```python
from build123d import *

# Parameters (mm, degrees)
F2_R           = 12.6873
F3_DEPTH       = 1.524
F4_R           = 10.16
F5_DEPTH       = 25.4
F7_ANGLE       = 10
F8_W           = 12.7
F8_H           = 2.5441443902
F9_ANGLE_BACK  = 5
F9_ANGLE       = 20
F10_W          = 12.7
F10_H          = 2.5441443902
F11_ANGLE_BACK = 5
F11_ANGLE      = 20


with BuildPart() as f1:
    # F0 (on Front) → F1 (revolve)
    with BuildSketch(Plane.XZ):
        with BuildLine():
            Line((-13.97, 0), (-12.7, 0))
            Line((-12.7, 0), (-12.7, 5.76834))
            ThreePointArc((-12.7, 5.76834), (-12.5140128061, 6.2173528061), (-12.065, 6.40334))
            Line((-12.065, 6.40334), (0, 6.40334))
            Line((0, 6.40334), (0, 8.43534))
            Line((0, 8.43534), (-12.0142573769, 8.43534))
            ThreePointArc((-12.0142573769, 8.43534), (-13.3560582498, 7.8825956776), (-13.9192, 6.5451252153))
            Line((-13.9192, 6.5451252153), (-13.97, 0))
        make_face()
    revolve(axis=Axis((0, 0, 7.41934), (0, 0, 1)))

    # F2 (on face) → F3 (cut)
    with BuildSketch(Plane.XY.offset(8.43534)):
        Circle(F2_R)
    extrude(amount=-F3_DEPTH, mode=Mode.SUBTRACT)

    # F4 (on face) → F5 (cut)
    with BuildSketch(Plane.XY.offset(6.91134)):
        Circle(F4_R)
    extrude(amount=-F5_DEPTH, mode=Mode.SUBTRACT)

    # F6 (on Right) → F7 (revolve)
    with BuildSketch(Plane.YZ):
        with BuildLine():
            add(Edge.make_bspline(
                [(-12.7, 2.54), (-12.3650313684, 2.0936619038), (-12.0236620945, 1.3279431517), (-12.3556444426, 0.3304517928), (-12.7, 0)],
                knots=[0, 0, 0, 0, 0.5, 1, 1, 1, 1], degree=3))
            Line((-12.7, 2.54), (-12.7, 0))
        make_face()
        with BuildLine():
            Line((12.7, 0), (12.7, 2.54))
            add(Edge.make_bspline(
                [(12.7, 2.54), (12.4156702788, 2.2468428115), (11.9749216364, 1.2698282605), (12.4024864485, 0.2935006674), (12.7, 0)],
                knots=[0, 0, 0, 0, 0.5, 1, 1, 1, 1], degree=3))
        make_face()
    revolve(axis=Axis((0, 0, 2.8421400978), (0, 0, 1)), revolution_arc=F7_ANGLE)

    # F8 (on Right) → F9 (revolve, cut)
    with BuildSketch(Plane.YZ, mode=Mode.PRIVATE) as f9_sk:
        with Locations((6.35, 7.0404121951)):
            Rectangle(F8_W, F8_H)
    revolve(f9_sk.sketch.rotate(Axis((0, 0, 7.0404121951), (0, 0, 1)), -F9_ANGLE_BACK), axis=Axis((0, 0, 7.0404121951), (0, 0, 1)), revolution_arc=F9_ANGLE, mode=Mode.SUBTRACT)

    # F10 (on Right) → F11 (revolve, cut)
    with BuildSketch(Plane.YZ, mode=Mode.PRIVATE) as f11_sk:
        with Locations((-6.35, 7.0404121951)):
            Rectangle(F10_W, F10_H)
    revolve(f11_sk.sketch.rotate(Axis((0, 0, 7.0404121951), (0, 0, 1)), -F11_ANGLE_BACK), axis=Axis((0, 0, 7.0404121951), (0, 0, 1)), revolution_arc=F11_ANGLE, mode=Mode.SUBTRACT)


solid = f1.part
```
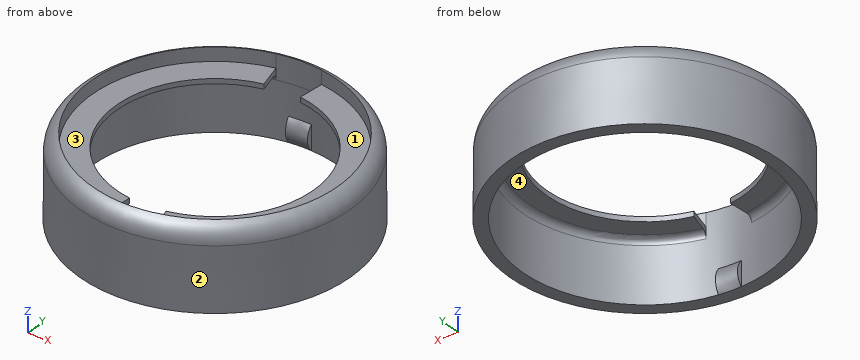
Read the model definition and answer for the solid it produces. Units are mm, in the model's axes. Face numbers are marked on the shaded views. A direction names the side the tool comes from. Coordinates: 2 decimals unless noted, no trailing zeros. Loops run counter-clockwise (first coordinate to the right, second up) from the corner with the lowest first, then second, coordinate; pieces in that order, holes last. Notation, with made-up numbers: (-4.5, 14) - (43.5, 14) arc R13 cw to (43.5, 32) - close; hole circle Ø5 at (0, 1.5). An arc over 180 degrees is marked (long way). Answer in a Markdown table with one row per item.
1. Find section A-A, the plane z = 7.5. Write down the section's boundary in (x, y) (3 decimals), then the cut area to 3 significant figures.
Conclusion:
| item | result |
|---|---|
| outline | circle Ø27.308 at (0, 0); hole (-3.287, 12.267) - (-3.284, 12.255) arc R12.687 ccw to (-1.106, -12.639) - (-1.107, -12.652) arc R12.7 ccw to (3.287, -12.267) - (3.284, -12.255) arc R12.687 ccw to (1.106, 12.639) - (1.107, 12.652) arc R12.7 ccw to start |
| area | 79.9 mm² |
2. Straight lines are drawn through the part: line 1 (X direction, y = 0, z = 6.5); line 2 (Y direction, x = 0, z = 5.75); line 3 (X direction, y = -0.5, z = 4.5). For each, find the intervals that lie inside material, in ascending order.
Conclusion:
| item | result |
|---|---|
| line 1 | x = -13.92 to -10.16, 10.16 to 13.92 |
| line 2 | y = -13.93 to -12.7, 12.7 to 13.93 |
| line 3 | x = -13.93 to -12.69, 12.69 to 13.93 |
3. Determine the mould class of the marked faces 1 and 2 for opening direction Y: +Y half, -Y half, draft (parallel to the pull), parting line (faces both ways), or undercut.
Conclusion:
| item | result |
|---|---|
| face 1 | undercut |
| face 2 | parting line |
4. Given pin 1 (12.5 mm diameter, centred on x = 4, y = 4.5, fed in from -Z); pin 2 (2 mm diameter, centred on y = -11, z = 1.5, fed in from +X); pin 3 (1 mm diameter, centred on y = -6.5, z = 7, fed in from -X), each flat-ended and moving along its own axis, determine where each tip first touches the part or whether it passes through.
Conclusion:
| item | result |
|---|---|
| pin 1 | stops at z = 6.37 |
| pin 2 | stops at x = 9.74 |
| pin 3 | stops at x = -12.52 |
5. Which of the six approach directions +Z, -Z, +X, -X, +Y, -Y give full straight-line access (tool end or side, diameter ignored) to the marked faces 3 and 4?
Conclusion:
| item | result |
|---|---|
| face 3 | +Z |
| face 4 | -Z |
